Source: CAD feature listing. Evaluate the final solid. Frame: model axes, mm. A direction names the side the tool comes from. Round coordinates to 2 decimals unless told otherwise and drop trailing zeros. Write each loop counter-clockwise with the first axis right and the second up, starting at its lowest first coordinate (ties: lowest second). Pieces come first, ordered by that corner, then holes.
from build123d import *

# Parameters (mm, degrees)
EXTRUDE001_DEPTH = 24.5
EXTRUDE_DEPTH    = 46
FILLET001_R      = 1


with BuildPart() as extrude001:
    # Sketch002 (on Sketch) → Extrude001 (new body, symmetric)
    with BuildSketch(Plane(origin=(0, 0, 0), x_dir=(0, 0, 1), z_dir=(1, 0, 0))):
        Polygon((0, 0), (0, -4), (68, -4), (80, -4), (80, 0), (76, 0), (74, -2), (70, -2), (68, 0), align=None)
    extrude(amount=EXTRUDE001_DEPTH, both=True)


with BuildPart() as bin_holder:
    # Sketch001 → Extrude (new body)
    with BuildSketch(Plane.XZ):
        Polygon((24.5, 0), (-24.5, 0), (-24.5, 80), (-22.5, 81.154701), (-20.5, 80), (-20.5, 76), (-22.5, 74), (-22.5, 70), (-20.5, 68), (-20.5, 4), (20.5, 4), (20.5, 68), (22.5, 70), (22.5, 74), (20.5, 76), (20.5, 80), (22.5, 81.154701), (24.5, 80), align=None)
    extrude(amount=EXTRUDE_DEPTH)


with BuildPart() as bin_holder_1:
    # Extrude placement: moved
    add(bin_holder.part.moved(Location((0, 2, 0))))

    # Fusion: union Extrude001
    add(extrude001.part)

    # Fillet001
    fillet001_edges = [bin_holder_1.edges().sort_by_distance(p)[0] for p in [
        (-20.5, -22, 4),
        (0, 0, 4),
        (20.5, -22, 4),
    ]]
    fillet(fillet001_edges, radius=FILLET001_R)


solid = bin_holder_1.part
1) Section query A-A on y = -6. Return the cut outline in (x, z).
Taken from the geometry:
outline: (-24.5, 0) - (24.5, 0) - (24.5, 80) - (22.5, 81.15) - (20.5, 80) - (20.5, 76) - (22.5, 74) - (22.5, 70) - (20.5, 68) - (20.5, 5) arc R1 cw to (19.5, 4) - (-19.5, 4) arc R1 cw to (-20.5, 5) - (-20.5, 68) - (-22.5, 70) - (-22.5, 74) - (-20.5, 76) - (-20.5, 80) - (-22.5, 81.15) - (-24.5, 80) - close
2) Reachability of faces 4 (the face through (20.5, -22, 78)), 5 (the face through (-21.5, -20.7, 69)), 6 (the face through (0, 2, 80)) from +Z, -Z, +X, -X, +Y, -Y: full face, straight path, thin tool, end or side. Return the list, or none.
Taken from the geometry:
face 4: +Z, -Y
face 5: -Y
face 6: +Z, +Y
3) Section query B-B on x = -1. Return the cut outline in (y, z).
Taken from the geometry:
outline: (-44, 0) - (4, 0) - (4, 80) - (0, 80) - (0, 76) - (2, 74) - (2, 70) - (0, 68) - (0, 5) arc R1 cw to (-1, 4) - (-44, 4) - close
4) Material intervals for line 1 (X direction, y = -13, z = 76.5); line 2 (Y direction, x = 10, z = 29.5); line 3 (Y direction, x = 7, z = 72), sorted ascending.
Taken from the geometry:
line 1: x = -24.5 to -20.5, 20.5 to 24.5
line 2: y = 0 to 4
line 3: y = 2 to 4
5) Contact query for flat-ended pins moving along their axis: P1, Ø3, axis at x = 10, z = 70, coming from the -Y side; P2, Ø12.5, axis at x = -6, z = 40, coming from the -Y side; P3, Ø2, axis at x = 7.5, y = 3, coming from the +Z side. Output: stop coordinate, or through.
Taken from the geometry:
P1: stops at y = 0.5
P2: stops at y = 0
P3: stops at z = 80
6) Section query C-C on z = 16.5. Return the cut outline in (x, y).
Taken from the geometry:
outline: (-24.5, -44) - (-20.5, -44) - (-20.5, 0) - (20.5, 0) - (20.5, -44) - (24.5, -44) - (24.5, 4) - (-24.5, 4) - close
7) Pull-direction query (X, two-part tool) for faces 1 (the face through (0, -22, 4)), 2 (the face through (-24.5, -20, 39)), 3 (the face through (22, -44, 35)); classes: released by +X, released by -X, zero draft, split by the parting line, or undercut.
Taken from the geometry:
face 1: undercut
face 2: released by -X
face 3: zero draft
